Read the model definition and answer for the solid it produces. Units are mm, in the model's axes. Face numbers are marked on the shaded views. A direction names the side the tool comes from. Coordinates: 2 decimals unless noted, no trailing zeros. Loops run counter-clockwise (first coordinate to the right, second up) from the corner with the lowest first, then second, coordinate; pieces in that order, holes last. Notation, with made-up numbers: (-21.75, 40) -> (27.25, 40) arc R23 ccw to (27.25, 66) -> close; hole circle Ø4 at (73.5, 3.5). An arc over 180 degrees is marked (long way). Answer in a Markdown table with one row per item.
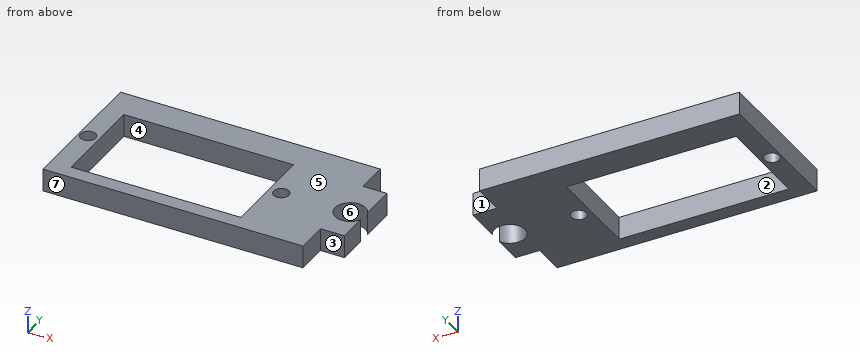
```python
from build123d import *

# Parameters (mm, degrees)
F0_R     = 1.1224142381
F0_W     = 22.305868566
F0_H     = 12.7213150263
F0_R_2   = 0.6302857898
F0_R_3   = 1.6961440054
F1_DEPTH = 3
F2_D     = 2
F3_D     = 2
F5_D     = 4


with BuildPart() as f1:
    # F0 (on Top) → F1 (new body)
    with BuildSketch(Plane.XY):
        Polygon((-29.121896252, 54.77469787), (-63.2777586579, 54.77469787), (-63.3072480559, 36.1355394125), (-29.121896252, 36.1355394125), (-29.121896252, 40.332082659), (-25.9702913463, 40.332082659), (-25.9702913463, 50.6002567708), (-29.121896252, 50.6002567708), align=None)
        with Locations((-62.0993860066, 44.8157414794)):
            Circle(F0_R, mode=Mode.SUBTRACT)
        with Locations((-49.5029501617, 44.4138646126)):
            Rectangle(F0_W, F0_H, mode=Mode.SUBTRACT)
        with Locations((-36.7128923535, 44.8157414794)):
            Circle(F0_R_2, mode=Mode.SUBTRACT)
        with Locations((-29.121896252, 45.4661697149)):
            Circle(F0_R_3, mode=Mode.SUBTRACT)
        with Locations((-29.121896252, 45.4661697149)):
            Circle(F0_R_3)
        with Locations((-62.0993860066, 44.8157414794)):
            Circle(F0_R)
        with Locations((-36.7128923535, 44.8157414794)):
            Circle(F0_R_2)
    extrude(amount=F1_DEPTH)

    # F2 (through all)
    with Locations(Plane(origin=(0, 0, 0), x_dir=(1, 0, 0), z_dir=(0, 0, -1))):
        with Locations((-62.0993860066, -44.8157414794)):
            Hole(F2_D / 2)

    # F3 (through all)
    with Locations(Plane(origin=(0, 0, 0), x_dir=(1, 0, 0), z_dir=(0, 0, -1))):
        with Locations((-36.7128923535, -44.8157414794)):
            Hole(F3_D / 2)

    # F5 (through all)
    with Locations(Plane.XY.offset(3)):
        with Locations((-27.7918130159, 45.0828969479)):
            Hole(F5_D / 2)


solid = f1.part
```
1. A cutting plane is placed at B-B on y = 50.25. Give the vertices of the cut face in (x, z), and give its area (3 significant figures).
A:
| item | result |
|---|---|
| outline | (-63.28, 0) -> (-60.66, 0) -> (-60.66, 3) -> (-63.28, 3) -> close; (-38.35, 0) -> (-25.97, 0) -> (-25.97, 3) -> (-38.35, 3) -> close |
| area | 45.0 mm2 |
2. A cutting plane is placed at D-D on y = 52.75. Give the vertices of the cut face in (x, z), and give its area (3 significant figures).
A:
| item | result |
|---|---|
| outline | (-63.28, 0) -> (-29.12, 0) -> (-29.12, 3) -> (-63.28, 3) -> close |
| area | 102 mm2 |
3. A tool of negligible diameter and unlimited length cuts with its end or side. For the marked faces 1, 2 and 3, from which of +Z, -Z, +X, -X, +Y, -Y can it reach the whole face along a straight path? Write none if from no direction.
A:
| item | result |
|---|---|
| face 1 | +Z, -Z, +X, +Y |
| face 2 | +Z, -Z |
| face 3 | +Z, -Z, +X, -Y |
4. The mould has two halves that part along Y. Classify the marked faces 4, 5, 6 and 7: pulls with the +Y half, pulls with the -Y half, needs draft (parallel to the pull), parting line crosses it, or undercut.
A:
| item | result |
|---|---|
| face 4 | undercut |
| face 5 | needs draft |
| face 6 | undercut |
| face 7 | pulls with the -Y half |
5. Find the intervals of material crossed by probe 1 along X at (y, z) = (39.5, 2.3); probe 2 along Y at (x, z) = (-38.5, 1.35); probe 3 along X at (y, z) = (45.5, 2.2), in increasing order.
A:
| item | result |
|---|---|
| probe 1 | x = -63.3 to -60.66, -38.35 to -29.12 |
| probe 2 | y = 36.14 to 38.05, 50.77 to 54.77 |
| probe 3 | x = -63.29 to -62.83, -61.37 to -60.66, -38.35 to -37.44, -35.98 to -29.75 |
6. A cutting plane is placed at A-A on x = -57. Give the vertices of the cut face in (y, z).
A:
| item | result |
|---|---|
| outline | (36.14, 0) -> (38.05, 0) -> (38.05, 3) -> (36.14, 3) -> close; (50.77, 0) -> (54.77, 0) -> (54.77, 3) -> (50.77, 3) -> close |
7. A cutting plane is placed at C-C on z = 1.05. Give the vertices of the cut face in (x, y), and give its area (3 significant figures).
A:
| item | result |
|---|---|
| outline | (-63.31, 36.14) -> (-29.12, 36.14) -> (-29.12, 40.33) -> (-25.97, 40.33) -> (-25.97, 44.26) arc R2 cw (long way) to (-25.97, 45.91) -> (-25.97, 50.6) -> (-29.12, 50.6) -> (-29.12, 54.77) -> (-63.28, 54.77) -> close; hole circle Ø2 at (-62.1, 44.82); hole (-60.66, 38.05) -> (-38.35, 38.05) -> (-38.35, 50.77) -> (-60.66, 50.77) -> close; hole circle Ø2 at (-36.71, 44.82) |
| area | 367 mm2 |
8. Given pin 1 Ø5 at (x, y) = (-46.5, 47) entering from -Z; pin 2 Ø1.5 at (x, z) = (-28, 1) entering from +Y, each flat-ended and moving along its own axis, determine where each tip first touches the part or whether it passes through.
A:
| item | result |
|---|---|
| pin 1 | passes through |
| pin 2 | stops at y = 50.6 |
